Build history of the part. All positions in model axes, mm. Face numbers are marked on the shaded views. A direction names the side the tool comes from. Round coordinates to 2 decimals unless told otherwise and drop trailing zeros. Loops run counter-clockwise (first coordinate to the right, second up) from the corner with the lowest first, then second, coordinate; pieces in that order, holes last.
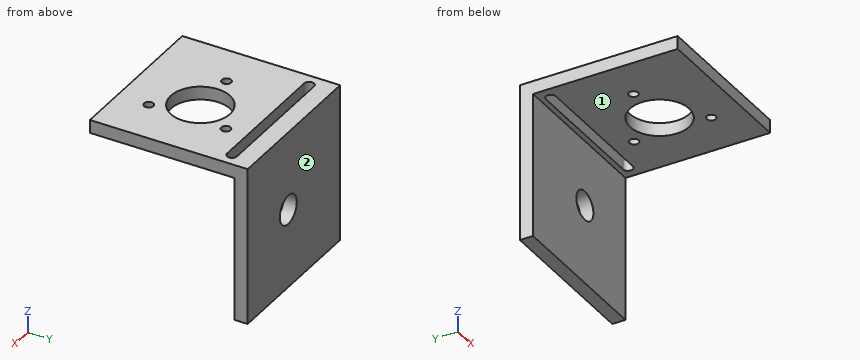
from build123d import *

# Parameters (mm, degrees)
BOSS_EXTRUDE1_DEPTH  = 76.2
SKETCH2_R            = 14.2875
CUT_EXTRUDE1_DEPTH   = 132.982271537
M4_CLEARANCE_HOLE1_D = 4.5
CUT_EXTRUDE2_REACH   = 130.421
SKETCH6_R            = 7
CUT_EXTRUDE3_DEPTH   = 129.420802443


with BuildPart() as part:
    # Sketch1 → Boss-Extrude1 (new body)
    with BuildSketch(Plane(origin=(0, 0, 0), x_dir=(0, 0, -1), z_dir=(1, 0, 0))):
        Polygon((-6.35, 76.2), (69.85, 76.2), (69.85, 69.85), (0, 69.85), (0, 0), (-6.35, 0), align=None)
    extrude(amount=BOSS_EXTRUDE1_DEPTH)

    # Sketch2 → Cut-Extrude1 (cut, through all)
    with BuildSketch(Plane.XY.offset(6.35)):
        with Locations((42.729606228, 33.762)):
            Circle(SKETCH2_R)
    extrude(amount=-CUT_EXTRUDE1_DEPTH, mode=Mode.SUBTRACT)

    # M4 Clearance Hole1 (through all)
    with Locations(Plane.XY.offset(6.35)):
        with Locations((53.479606228, 52.381546181), (21.229606228, 33.762), (53.479606228, 15.142453819)):
            Hole(M4_CLEARANCE_HOLE1_D / 2)

    # Sketch6 → Cut-Extrude2 (cut, up to next)
    with BuildSketch(Plane(origin=(0, 76.2, 0), x_dir=(1, 0, 0), z_dir=(0, 1, 0)), mode=Mode.PRIVATE) as cut_extrude2_sk1:
        with Locations(Location((42.729614414, 31.75, 0), (0, 0, 270))):
            Circle(SKETCH6_R)
    cut_extrude2_tool1 = extrude(cut_extrude2_sk1.sketch, amount=-CUT_EXTRUDE2_REACH, mode=Mode.PRIVATE) & part.part
    add(cut_extrude2_tool1.solids().sort_by_distance((42.729614, 76.2, -31.75))[0], mode=Mode.SUBTRACT)

    # Sketch7 → Cut-Extrude3 (cut, through all)
    with BuildSketch(Plane(origin=(0, 0, 0), x_dir=(-1, 0, 0), z_dir=(0, 0, -1))):
        with BuildLine():
            Line((-69.85, 67.31), (-6.35, 67.31))
            ThreePointArc((-6.35, 67.31), (-3.96875, 64.92875), (-6.35, 62.5475))
            Line((-6.35, 62.5475), (-69.85, 62.5475))
            ThreePointArc((-69.85, 62.5475), (-72.23125, 64.92875), (-69.85, 67.31))
        make_face()
    extrude(amount=-CUT_EXTRUDE3_DEPTH, mode=Mode.SUBTRACT)


solid = part.part
(1) Slice it at A-A on z = -31.75. List the corners of the cut face in (x, y), plus the area to 3 significant figures.
Responses:
outline: (0, 69.85) - (35.73, 69.85) - (35.73, 76.2) - (0, 76.2) - close; (49.73, 69.85) - (76.2, 69.85) - (76.2, 76.2) - (49.73, 76.2) - close
area: 395 mm2
(2) Slice it at B-B on x = 68. List the corners of the cut face in (y, z), plus the area to 3 significant figures.
Responses:
outline: (0, 0) - (62.55, 0) - (62.55, 6.35) - (0, 6.35) - close; (67.31, 0) - (69.85, 0) - (69.85, -69.85) - (76.2, -69.85) - (76.2, 6.35) - (67.31, 6.35) - close
area: 897 mm2
(3) Slice it at C-C on y = 44.5. List the corners of the cut face in (x, z), plus the area to 3 significant figures.
Responses:
outline: (0, 0) - (33.3, 0) - (33.3, 6.35) - (0, 6.35) - close; (52.15, 0) - (76.2, 0) - (76.2, 6.35) - (52.15, 6.35) - close
area: 364 mm2
(4) Pin check, flat tips, straight feed: P1, Ø5, axis at x = 53.48, y = 15.14, coming from the -Z side; P2, Ø2, axis at x = 27.5, z = -30, coming from the -Y side. Stop position of each tip, or through.
Responses:
P1: stops at z = 0
P2: stops at y = 69.85
(5) Slice it at D-D on x = 21. List the corners of the cut face in (y, z).
Responses:
outline: (0, 0) - (31.52, 0) - (31.52, 6.35) - (0, 6.35) - close; (36, 0) - (62.55, 0) - (62.55, 6.35) - (36, 6.35) - close; (67.31, 0) - (69.85, 0) - (69.85, -69.85) - (76.2, -69.85) - (76.2, 6.35) - (67.31, 6.35) - close
(6) Probe line 1 (Y direction, x = 61.5, z = 2); line 2 (Y direction, x = 52, z = -19); line 3 (Z direction, x = 63, y = 40.5). List the from-to ranges inside material, lowest first.
Responses:
line 1: y = 0 to 62.55, 67.31 to 76.2
line 2: y = 69.85 to 76.2
line 3: z = 0 to 6.35
(7) Which spindle directions (+Z, -Z, +X, -X, +Y, -Y) get a long thin tool onto all of the face, cutting with end or side? Do the marked faces 1 and 2. Say none if no direction does.
Responses:
face 1: -Z, +X, -X, -Y
face 2: +Z, -Z, +X, -X, +Y
